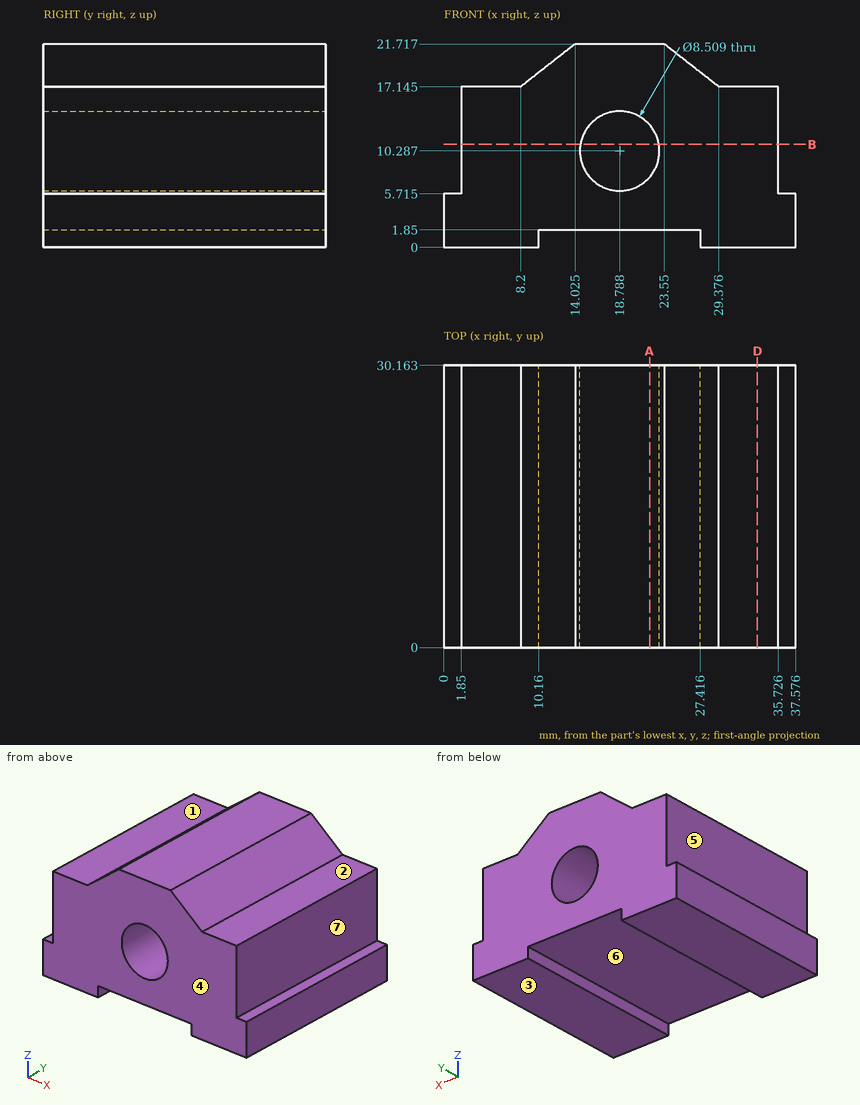
For this review, use the dimensioned drawing (mm, ordinates from the lowest corner) and the shaded views. A direction names the side the tool comes from. Round coordinates to 2 decimals unless told otherwise and drop trailing zeros. Write each loop counter-clockwise with the first axis right and the second up, starting at its lowest first coordinate (ties: lowest second). Pieces come first, ordered by that corner, then holes. Notation, with made-up numbers: M 55.25,44 L 90.25,44 A22 cw 90.25,53 Z; hole C 26.25,52 d3. An arc over 180 degrees is marked long. Use CSV: the item, a comma, the result in double quotes. Start each with the question number.
(1) Tool access review of the marked faces 1, 2 and 3: name each direction out of +Z, -Z, +X, -X, +Y, -Y from which nothing blocks a thin tool from reaching the whole face with its end or side.
(2) We need section D-D, the plane x = 33.5. State the section outline as (y, z) points (1 decimal).
(3) We need section A-A, the plane x = 22. State the section outline as (y, z) points.
(4) We need section B-B, the plane z = 11. State the section outline as (x, y) points, then the cut area to 3 significant figures.
(5) The part is to be moulded in two halves that separate along X. For the marked faces 4, 5, 6 and 7, say which applies: +X half, -X half, draft (parallel to the pull), parting line (faces both ways), or undercut.
(6) For line 1 along X through (y, z) = (19, 1.25) (1 decimal); line 2 along Z through (x, y) = (5, 9) (1 decimal); line 3 along X through (y, z) = (15.5, 16.75), list the stretches that pass through material, from the lowest coordinate up.
(7) Clearance check with flat-ended pins moving along their axes: P1, Ø2, axis at x = 1, y = 13, coming from the +Z side (1 decimal); P2, Ø3.5, axis at y = 16.5, z = 11, coming from the +X side; P3, Ø5.5, axis at y = 13, z = 11, coming from the -X side; P4, Ø7.5, axis at x = 18.79, z = 10.29, coming from the -Y side. State where each tip first meets the part, or that it passes through.
Findings:
1,face 1,"+Z, -X, +Y, -Y"
1,face 2,"+Z, +X, +Y, -Y"
1,face 3,"-Z, +X, -X, +Y, -Y"
2,outline,"M 0,0 L 30.2,0 L 30.2,17.1 L 0,17.1 Z"
3,outline,"M 0,1.85 L 30.16,1.85 L 30.16,7.5 L 0,7.5 Z; M 0,13.08 L 30.16,13.08 L 30.16,21.72 L 0,21.72 Z"
4,outline,"M 1.85,0 L 14.59,0 L 14.59,30.16 L 1.85,30.16 Z; M 22.98,0 L 35.73,0 L 35.73,30.16 L 22.98,30.16 Z"
4,area,"769 mm^2"
5,face 4,"draft"
5,face 5,"-X half"
5,face 6,"undercut"
5,face 7,"+X half"
6,line 1,"0 to 10.2, 27.4 to 37.6"
6,line 2,"0 to 17.1"
6,line 3,"1.85 to 35.73"
7,P1,"z = 17.1"
7,P2,"x = 35.73"
7,P3,"x = 1.85"
7,P4,"through"
